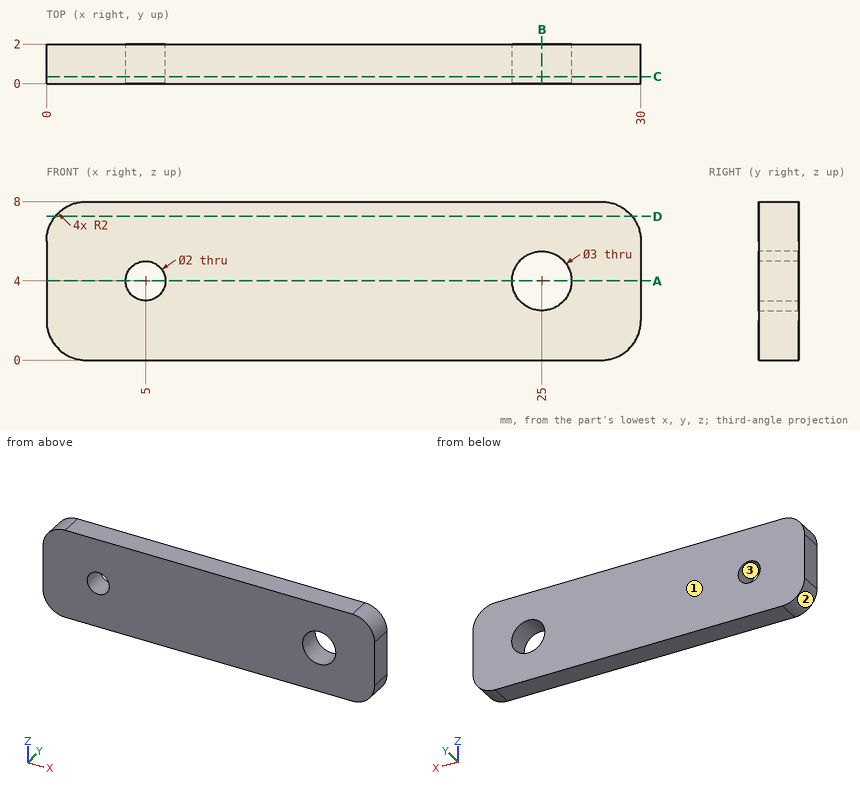
Source: three-view drawing plus pictorial views. Frame: mm from the lowest corner of the part. Round coordinates to 2 decimals unless told otherwise and drop trailing zeros. Loops run counter-clockwise (first coordinate to the right, second up) from the corner with the lowest first, then second, coordinate; pieces in that order, holes last.
1. Section query A-A on z = 4. Output: boundary loops of the cut face in (x, y).
2. Section query C-C on y = 0.35. Output: boundary loops of the cut face in (x, z).
3. Ray query, L1, parallel to X at y = 1.4, z = 4; L2, parallel to Z at x = 24.5, y = 1.25; L3, parallel to X at y = 1.35, z = 3.5. Return the intervals inside material, ascending.
4. Section query D-D on z = 7.25. Output: boundary loops of the cut face in (x, y).
5. Contact query for a flat-ended pin moving along its axis: pin 1 (2.5 mm diameter, centred on x = 25, z = 4, fed in from +Y). Output: stop coordinate, or through.
6. Mould query, pull axis X, two halves, no side actions, for the marked faces 1, 2 and 3. Classes: released by +X, released by -X, zero draft, split by the parting line, or undercut.
7. Section query B-B on x = 25. Output: boundary loops of the cut face in (y, z), and give its area (3 significant figures).
Answers below:
1. outline: (0, 0) - (4, 0) - (4, 2) - (0, 2) - close; (6, 0) - (23.5, 0) - (23.5, 2) - (6, 2) - close; (26.5, 0) - (30, 0) - (30, 2) - (26.5, 2) - close
2. outline: (0, 2) arc R2 ccw to (2, 0) - (28, 0) arc R2 ccw to (30, 2) - (30, 6) arc R2 ccw to (28, 8) - (2, 8) arc R2 ccw to (0, 6) - close; hole circle Ø2 at (5, 4); hole circle Ø3 at (25, 4)
3. L1: x = 0 to 4, 6 to 23.5, 26.5 to 30
3. L2: z = 0 to 2.59, 5.41 to 8
3. L3: x = 0 to 4.13, 5.87 to 23.59, 26.41 to 30
4. outline: (0.44, 0) - (29.56, 0) - (29.56, 2) - (0.44, 2) - close
5. pin 1: passes through
6. face 1: zero draft
6. face 2: released by -X
6. face 3: undercut
7. outline: (0, 0) - (2, 0) - (2, 2.5) - (0, 2.5) - close; (0, 5.5) - (2, 5.5) - (2, 8) - (0, 8) - close
7. area: 10.0 mm2
